```python
from build123d import *

# Parameters (mm, degrees)
SKETCH1_W           = 10
SKETCH1_H           = 5
BOSS_EXTRUDE1_DEPTH = 50
SKETCH2_R           = 2
CUT_EXTRUDE1_DEPTH  = 10


with BuildPart() as part:
    # Sketch1 → Boss-Extrude1 (new body)
    with BuildSketch(Plane.XY):
        Rectangle(SKETCH1_W, SKETCH1_H)
    extrude(amount=BOSS_EXTRUDE1_DEPTH)

    # Sketch2 → Cut-Extrude1 (cut)
    with BuildSketch(Plane(origin=(0, 2.5, 0), x_dir=(1, 0, 0), z_dir=(0, 1, 0))):
        with Locations((0, -43)):
            Circle(SKETCH2_R)
        with Locations((0, -25)):
            Circle(SKETCH2_R)
        with Locations((0, -7)):
            Circle(SKETCH2_R)
    extrude(amount=-CUT_EXTRUDE1_DEPTH, mode=Mode.SUBTRACT)


solid = part.part
```
Check sheet for the modelled part. Datum: model origin and axes. Units: mm. Give positions to 0.01 mm unless a question says otherwise; leave off trailing zeros. Write each loop counter-clockwise with the first axis right and the second up, starting at its lowest first coordinate (ties: lowest second). Pieces come first, ordered by that corner, then holes. Notation, with made-up numbers: (80.25, 66) - (138.25, 66) arc R18 cw to (138.25, 81) - close; hole circle Ø11 at (76.5, -13.75). An arc over 180 degrees is marked (long way). Answer as a JSON object with one key per item and string values. Group by question number.
1) Sectioned sample at C-C (z = 43). Record the cut outline in (x, y).
2) Sectioned sample at B-B (x = 0). Record the cut outline in (y, z).
3) Release check for a two-part mould opening along X. For faces 1 (the face through (0.923, 0.035, 26.774)), 2 (the face through (0, 0, 45)), 3 (the face through (0, 0, 0)), 4 (the face through (5, 0, 25)) record: pulls with the +X half, pulls with the -X half, needs draft (parallel to the pull), parting line crosses it, or undercut.
4) Depth check by flat-ended pin: P1, Ø4.5, axis at x = 0, z = 7, coming from the +Y side. Enter the tip coordinate at first touch or a pass-through.
5) Thickness scan on probe 1 along Z at (x, y) = (0, 0.05); probe 2 along Z at (x, y) = (-1.5, 1.2); probe 3 along X at (y, z) = (-0.15, 43). Record the ranges inside material, lowest first. Write a range as from..to.
6) Sectioned sample at A-A (y = -2). Record the cut outline in (x, z).
Geometry results:
{
 "1": {"outline": "(-5, -2.5) - (-2, -2.5) - (-2, 2.5) - (-5, 2.5) - close; (2, -2.5) - (5, -2.5) - (5, 2.5) - (2, 2.5) - close"},
 "2": {"outline": "(-2.5, 0) - (2.5, 0) - (2.5, 5) - (-2.5, 5) - close; (-2.5, 9) - (2.5, 9) - (2.5, 23) - (-2.5, 23) - close; (-2.5, 27) - (2.5, 27) - (2.5, 41) - (-2.5, 41) - close; (-2.5, 45) - (2.5, 45) - (2.5, 50) - (-2.5, 50) - close"},
 "3": {"face 1": "undercut", "face 2": "undercut", "face 3": "needs draft", "face 4": "pulls with the +X half"},
 "4": {"P1": "stops at y = 2.5"},
 "5": {"probe 1": "z = 0..5, 9..23, 27..41, 45..50", "probe 2": "z = 0..5.68, 8.32..23.68, 26.32..41.68, 44.32..50", "probe 3": "x = -5..-2, 2..5"},
 "6": {"outline": "(-5, 0) - (5, 0) - (5, 50) - (-5, 50) - close; hole circle Ø4 at (0, 7); hole circle Ø4 at (0, 25); hole circle Ø4 at (0, 43)"}
}
